Can you work these out from the model? Positions are in its coordinate system, mm. Round coordinates to 2 decimals unless told otherwise and drop trailing zeros. Order: outer loops, then holes, each group sorted by start corner. A loop starts at its lowest first (then second) coordinate and runs counter-clockwise, first axis right, second up. Notation, with made-up numbers: (48.25, 65.5) -> (84.25, 65.5) arc R29 ccw to (84.25, 90.5) -> close; hole circle Ø5 at (69, 69.25). An arc over 180 degrees is marked (long way). One line per item, written item: value.
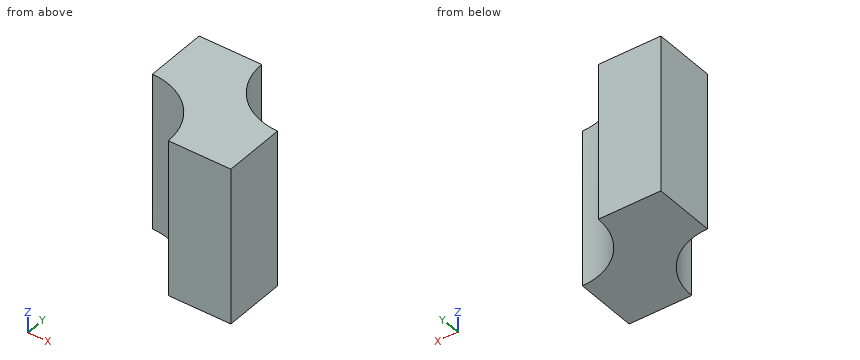
```python
from build123d import *

# Parameters (mm, degrees)
BOSS_EXTRUDE1_DEPTH = 25


with BuildPart() as part:
    # Sketch1 → Boss-Extrude1 (new body)
    with BuildSketch(Plane.XY):
        with BuildLine():
            Line((-20, 10), (-20, 20))
            Line((-20, 20), (-10, 20))
            ThreePointArc((-10, 20), (-7.071067812, 12.928932188), (0, 10))
            Line((0, 10), (0, 0))
            Line((0, 0), (-10, 0))
            ThreePointArc((-10, 0), (-12.928932188, 7.071067812), (-20, 10))
        make_face()
    extrude(amount=BOSS_EXTRUDE1_DEPTH)


solid = part.part
```
Q1. I want a section at A-A on z = 4.25. List the corners of the cut face in (x, y) for me, plus the area to 3 significant figures.
Answers below:
outline: (-20, 10) arc R10 cw to (-10, 0) -> (0, 0) -> (0, 10) arc R10 cw to (-10, 20) -> (-20, 20) -> close
area: 243 mm^2
Q2. I want a section at C-C on y = 12. List the corners of the cut face in (x, z) for me.
Answers below:
outline: (-20, 0) -> (-6, 0) -> (-6, 25) -> (-20, 25) -> close
Q3. Will this pin go through, and if not, where does the flat tip stop? pin 1 Ø3 at (x, y) = (-5, 15) entering from -Z.
Answers below:
pin 1: through
Q4. I want a section at B-B on x = -12. List the corners of the cut face in (y, z) for me.
Answers below:
outline: (6, 0) -> (20, 0) -> (20, 25) -> (6, 25) -> close
Q5. Please list where these lines run through material, in increasing order: line 1 along X through (y, z) = (15.25, 13.25); line 2 along Y through (x, z) = (-7.5, 6.25); line 3 along Y through (x, z) = (-1.25, 15.25).
Answers below:
line 1: -20 to -8.8
line 2: 0 to 13.39
line 3: 0 to 10.08
